Source: CAD feature listing. Evaluate the final solid. Frame: model axes, mm. A direction names the side the tool comes from. Round coordinates to 2 decimals unless told otherwise and drop trailing zeros. Order: outer loops, then holes, each group sorted by start corner. A loop starts at its lowest first (then second) coordinate and runs counter-clockwise, first axis right, second up. Notation, with made-up numbers: (41.25, -11) - (71.25, -11) arc R30 cw to (71.25, 18) - close; hole circle Ø4 at (17.25, -12.75). An arc over 180 degrees is marked (long way). Use one line per item in the form item = value. Start each with the question number.
Q1. Cut plane C-C, the plane z = 47. Return the cut outline in (x, y).
Q2. Draft query along X for faces 1 (the cylindrical face through (-17.3, 5.9, 37.7)), 2 (the flat face through (55.5, 6, 0)), 3 (the flat face through (-37.5, 6, 48)). Return one class per face: released by +X, released by -X, zero draft, split by the parting line, or undercut.
Q3. Set-up query: faces 4 (the cylindrical face through (-29.727, 8.082, 42.928)), 5 (the flat face through (-48, 6, 37.5)), 6 (the cylindrical face through (42.928, 8.082, -30.273)). Return all of +Z, -Z, +X, -X, +Y, -Y with unobstructed straight access to the full face (end or side cutting, diameter ignored); none if empty.
Q4. Cut plane D-D, the plane y = 10. Give the number of separate pieces and of enclosed holes in the cut face, and give its area (3 significant figures).
Q5. Ray query, line 1 (Z direction, x = -1, y = 9.5); line 2 (X direction, y = 2.5, z = -40); line 3 (Y direction, x = -30, z = -49). Return the intervals inside material, ascending. Write a range as [from, to].
Q6. Pin query (flat end, axial travel): pin 1 Ø3.5 at (y, z) = (4, -49.5) entering from -X; pin 2 Ø3.5 at (x, y) = (-49, 3.5) entering from +Z. Return the tip coordinate at first contact, or that it passes through.
Q7. Cut plane B-B, the plane x = 10. Return the cut outline in (y, z), and give its area (3 significant figures).
Q8. Cut plane A-A, the plane z = 0. Return the cut outline in (x, y).
from build123d import *

# Parameters (mm, degrees)
SKETCH_1_W               = 111
SKETCH_1_H               = 111
EXTRUDE_1_DEPTH          = 12
SKETCH_2_R               = 39
CUT_EXTRUDE_1_DEPTH      = 80.400881607
HOLE_WIZARD_M4_1_D       = 3.3
PATTERN_CIRCULAR_1_COUNT = 8
SKETCH_8_W               = 36
SKETCH_8_H               = 36
CUT_EXTRUDE_2_DEPTH      = 80.400881607
FILLET_1_R               = 5
CHAMFER_1_SIZE           = 2
HOLE_WIZARD_M5_1_REACH   = 126.681
HOLE_WIZARD_M5_1_BORE_R  = 2.1
HOLE_WIZARD_M5_2_REACH   = 126.681
HOLE_WIZARD_M5_2_BORE_R  = 2.1


with BuildPart() as part:
    # Sketch 1 → Extrude 1 (new body)
    with BuildSketch(Plane(origin=(0, 0, 0), x_dir=(1, 0, 0), z_dir=(0, 1, 0))):
        Rectangle(SKETCH_1_W, SKETCH_1_H)
    extrude(amount=EXTRUDE_1_DEPTH)

    # Sketch 2 → Cut-Extrude 1 (cut, through all)
    with BuildSketch(Plane(origin=(0, 12, 0), x_dir=(1, 0, 0), z_dir=(0, 1, 0))):
        with Locations(Location((0, 0, 0), (0, 0, 270))):
            Circle(SKETCH_2_R)
    extrude(amount=-CUT_EXTRUDE_1_DEPTH, mode=Mode.SUBTRACT)

    # Hole Wizard M4 _1 (through all)
    with Locations(Plane(origin=(0, 12, 0), x_dir=(1, 0, 0), z_dir=(0, 1, 0))):
        with Locations((-16.072704159, 38.802940365)):
            hole_wizard_m4_1 = Hole(HOLE_WIZARD_M4_1_D / 2)

    # Pattern Circular 1: Hole Wizard M4 _1 ×8 about axis
    pattern_circular_1_axis = Axis((0, 0, 0), (0, 1, 0))
    for i in range(1, PATTERN_CIRCULAR_1_COUNT):
        add(hole_wizard_m4_1.rotate(pattern_circular_1_axis, i * 360 / PATTERN_CIRCULAR_1_COUNT), mode=Mode.SUBTRACT)

    # Sketch 8 → Cut-Extrude 2 (cut, through all)
    with BuildSketch(Plane(origin=(0, 12, 0), x_dir=(1, 0, 0), z_dir=(0, 1, 0))):
        with Locations((-55.5, 55.5)):
            Rectangle(SKETCH_8_W, SKETCH_8_H)
        with Locations((55.5, 55.5)):
            Rectangle(SKETCH_8_W, SKETCH_8_H)
        with Locations((55.5, -55.5)):
            Rectangle(SKETCH_8_W, SKETCH_8_H)
        with Locations((-55.5, -55.5)):
            Rectangle(SKETCH_8_W, SKETCH_8_H)
    extrude(amount=-CUT_EXTRUDE_2_DEPTH, mode=Mode.SUBTRACT)

    # Fillet 1
    fillet_1_edges = [part.edges().sort_by_distance(p)[0] for p in [
        (-37.5, 6, 37.5),
        (37.5, 6, 37.5),
        (-37.5, 6, -37.5),
        (37.5, 6, -37.5),
    ]]
    fillet(fillet_1_edges, radius=FILLET_1_R)

    # Chamfer 1
    chamfer_1_edges = [part.edges().sort_by_distance(p)[0] for p in [
        (-55.5, 6, 37.5),
        (-37.5, 6, 55.5),
        (37.5, 6, 55.5),
        (55.5, 6, 37.5),
        (-37.5, 6, -55.5),
        (-55.5, 6, -37.5),
        (55.5, 6, -37.5),
        (37.5, 6, -55.5),
    ]]
    chamfer(chamfer_1_edges, length=CHAMFER_1_SIZE)

    # Hole Wizard M5 _1 bore → Hole Wizard M5 _1 (cut, up to next)
    with BuildSketch(Plane.ZY.offset(55.5), mode=Mode.PRIVATE) as hole_wizard_m5_1_sk1:
        with Locations((-30, 6)):
            Circle(HOLE_WIZARD_M5_1_BORE_R)
    hole_wizard_m5_1_tool1 = extrude(hole_wizard_m5_1_sk1.sketch, amount=-HOLE_WIZARD_M5_1_REACH, mode=Mode.PRIVATE) & part.part
    # Hole Wizard M5 _1 bore → Hole Wizard M5 _1 (cut, up to next)
    with BuildSketch(Plane.ZY.offset(55.5), mode=Mode.PRIVATE) as hole_wizard_m5_1_sk2:
        with Locations((30, 6)):
            Circle(HOLE_WIZARD_M5_1_BORE_R)
    hole_wizard_m5_1_tool2 = extrude(hole_wizard_m5_1_sk2.sketch, amount=-HOLE_WIZARD_M5_1_REACH, mode=Mode.PRIVATE) & part.part
    hole_wizard_m5_1_1 = hole_wizard_m5_1_tool1.solids().sort_by_distance((-55.5, 6, -30))[0]
    add(hole_wizard_m5_1_1, mode=Mode.SUBTRACT)
    hole_wizard_m5_1_2 = hole_wizard_m5_1_tool2.solids().sort_by_distance((-55.5, 6, 30))[0]
    add(hole_wizard_m5_1_2, mode=Mode.SUBTRACT)
    hole_wizard_m5_1 = hole_wizard_m5_1_1 + hole_wizard_m5_1_2  # Hole Wizard M5 _1 as one shape, for the pattern or mirror that repeats it

    # Hole Wizard M5 _2 bore → Hole Wizard M5 _2 (cut, up to next)
    with BuildSketch(Plane(origin=(0, 0, -55.5), x_dir=(-1, 0, 0), z_dir=(0, 0, -1)), mode=Mode.PRIVATE) as hole_wizard_m5_2_sk1:
        with Locations((-30, 6)):
            Circle(HOLE_WIZARD_M5_2_BORE_R)
    hole_wizard_m5_2_tool1 = extrude(hole_wizard_m5_2_sk1.sketch, amount=-HOLE_WIZARD_M5_2_REACH, mode=Mode.PRIVATE) & part.part
    # Hole Wizard M5 _2 bore → Hole Wizard M5 _2 (cut, up to next)
    with BuildSketch(Plane(origin=(0, 0, -55.5), x_dir=(-1, 0, 0), z_dir=(0, 0, -1)), mode=Mode.PRIVATE) as hole_wizard_m5_2_sk2:
        with Locations((30, 6)):
            Circle(HOLE_WIZARD_M5_2_BORE_R)
    hole_wizard_m5_2_tool2 = extrude(hole_wizard_m5_2_sk2.sketch, amount=-HOLE_WIZARD_M5_2_REACH, mode=Mode.PRIVATE) & part.part
    hole_wizard_m5_2_1 = hole_wizard_m5_2_tool1.solids().sort_by_distance((30, 6, -55.5))[0]
    add(hole_wizard_m5_2_1, mode=Mode.SUBTRACT)
    hole_wizard_m5_2_2 = hole_wizard_m5_2_tool2.solids().sort_by_distance((-30, 6, -55.5))[0]
    add(hole_wizard_m5_2_2, mode=Mode.SUBTRACT)
    hole_wizard_m5_2 = hole_wizard_m5_2_1 + hole_wizard_m5_2_2  # Hole Wizard M5 _2 as one shape, for the pattern or mirror that repeats it

    # Mirror 1: Hole Wizard M5 _2 across plane
    add(hole_wizard_m5_2.mirror(Plane.XY), mode=Mode.SUBTRACT)

    # Mirror 2: Hole Wizard M5 _1 mirrored; each copy of Hole Wizard M5 _1 runs up to whatever stops it at its own place
    mirror_2_before = part.part  # the part as the pattern finds it: every copy runs up to it
    mirror_2_hole_wizard_m5_1_long1 = extrude(hole_wizard_m5_1_sk1.sketch, amount=-HOLE_WIZARD_M5_1_REACH, mode=Mode.PRIVATE)
    mirror_2_hole_wizard_m5_1_long2 = extrude(hole_wizard_m5_1_sk2.sketch, amount=-HOLE_WIZARD_M5_1_REACH, mode=Mode.PRIVATE)
    mirror_2_hole_wizard_m5_1_tool1_1 = mirror_2_hole_wizard_m5_1_long1.mirror(Plane(origin=(0, 0, 0), x_dir=(0, 0, 1), z_dir=(1, 0, 0))) & mirror_2_before
    add(mirror_2_hole_wizard_m5_1_tool1_1.solids().sort_by_distance((55.5, 6, -30))[0], mode=Mode.SUBTRACT)
    mirror_2_hole_wizard_m5_1_tool2_1 = mirror_2_hole_wizard_m5_1_long2.mirror(Plane(origin=(0, 0, 0), x_dir=(0, 0, 1), z_dir=(1, 0, 0))) & mirror_2_before
    add(mirror_2_hole_wizard_m5_1_tool2_1.solids().sort_by_distance((55.5, 6, 30))[0], mode=Mode.SUBTRACT)


solid = part.part
Completed:
q1.outline = (-37.5, 0) - (37.5, 0) - (37.5, 12) - (-37.5, 12) - close; hole circle Ø4.2 at (-30, 6); hole circle Ø4.2 at (30, 6)
q2.face_1 = undercut
q2.face_2 = released by +X
q2.face_3 = released by -X
q3.face_4 = +Z
q3.face_5 = +Z, -X, +Y, -Y
q3.face_6 = +X
q4.separate_pieces = 1
q4.enclosed_holes = 9
q4.area = 6,180 mm2
q5.line_1 = [-55.5, -38.99], [38.99, 55.5]
q5.line_2 = [-38.17, -17.21], [-14.94, 14.94], [17.21, 38.17]
q5.line_3 = [0, 3.9], [8.1, 12]
q6.pin_1 = -37.5
q6.pin_2 = 37.5
q7.outline = (0, -55.5) - (12, -55.5) - (12, -37.7) - (0, -37.7) - close; (0, 37.7) - (12, 37.7) - (12, 55.5) - (0, 55.5) - close
q7.area = 427 mm2
q8.outline = (-55.5, 0) - (-39, 0) - (-39, 12) - (-55.5, 12) - close; (39, 0) - (55.5, 0) - (55.5, 12) - (39, 12) - close
